Source: CAD feature listing. Evaluate the final solid. Frame: model axes, mm. Give positions to 0.01 mm unless a question says otherwise; leave off trailing zeros. Loops run counter-clockwise (first coordinate to the right, second up) from the corner with the lowest first, then second, coordinate; pieces in that order, holes last. Notation, with made-up numbers: (-2.5, -32) -> (5.5, -32) arc R16 ccw to (5.5, -19) -> close; hole circle Ø10 at (-37.75, 23). An arc over 180 degrees is marked (long way). Put each result on its own line as item: value.
```python
from build123d import *

# Parameters (mm, degrees)
SKETCH2_W           = 170
SKETCH2_H           = 220
SKETCH2_R           = 2.6
SKETCH2_R_2         = 1
SKETCH2_R_3         = 20
BOSS_EXTRUDE1_DEPTH = 3.175


with BuildPart() as part:
    # Sketch2 → Boss-Extrude1 (new body)
    with BuildSketch(Plane(origin=(0, 0, 0), x_dir=(1, 0, 0), z_dir=(0, 1, 0))):
        Rectangle(SKETCH2_W, SKETCH2_H)
        with Locations((-75, 100)):
            Circle(SKETCH2_R, mode=Mode.SUBTRACT)
        with Locations((75, 100)):
            Circle(SKETCH2_R, mode=Mode.SUBTRACT)
        with Locations((75, -100)):
            Circle(SKETCH2_R, mode=Mode.SUBTRACT)
        with Locations((-75, -100)):
            Circle(SKETCH2_R, mode=Mode.SUBTRACT)
        with Locations((-6.954545455, 9)):
            Circle(SKETCH2_R_2, mode=Mode.SUBTRACT)
        with Locations((6.954545455, 9)):
            Circle(SKETCH2_R_2, mode=Mode.SUBTRACT)
        with Locations((6.954545455, -9)):
            Circle(SKETCH2_R_2, mode=Mode.SUBTRACT)
        with Locations((-6.954545455, -9)):
            Circle(SKETCH2_R_2, mode=Mode.SUBTRACT)
        with Locations((0, -48.117139718)):
            Circle(SKETCH2_R_3, mode=Mode.SUBTRACT)
    extrude(amount=BOSS_EXTRUDE1_DEPTH)


solid = part.part
```
(1) Section D-D on y = 1.95. Give the number of separate pieces and of enclosed holes in the cut face, then the cut area to 3 significant figures.
Calculated:
separate pieces: 1
enclosed holes: 9
area: 36,000 mm²
(2) Section A-A on x = -75. Return loops of the section in (y, z) (3 decimals).
Calculated:
outline: (0, -110) -> (3.175, -110) -> (3.175, -102.6) -> (0, -102.6) -> close; (0, -97.4) -> (3.175, -97.4) -> (3.175, 97.4) -> (0, 97.4) -> close; (0, 102.6) -> (3.175, 102.6) -> (3.175, 110) -> (0, 110) -> close
(3) Line query: probe 1 along X at (y, z) = (1.55, 100); probe 2 along Z at (x, y) = (75, 1.2); probe 3 along X at (y, z) = (1.2, 9). Output: solid intervals per line, ascending. Write a range as from..to.
Calculated:
probe 1: x = -85..-77.6, -72.4..72.4, 77.6..85
probe 2: z = -110..-102.6, -97.4..97.4, 102.6..110
probe 3: x = -85..-7.95, -5.95..5.95, 7.95..85
(4) Section B-B on z = 100. Return loops of the section in (x, y) (3 decimals).
Calculated:
outline: (-85, 0) -> (-77.6, 0) -> (-77.6, 3.175) -> (-85, 3.175) -> close; (-72.4, 0) -> (72.4, 0) -> (72.4, 3.175) -> (-72.4, 3.175) -> close; (77.6, 0) -> (85, 0) -> (85, 3.175) -> (77.6, 3.175) -> close
(5) Section C-C on x = 0. Return loops of the section in (y, z) (3 decimals).
Calculated:
outline: (0, -110) -> (3.175, -110) -> (3.175, 28.117) -> (0, 28.117) -> close; (0, 68.117) -> (3.175, 68.117) -> (3.175, 110) -> (0, 110) -> close
(6) Draft query along X for faces 1 (the cylindrical face through (73.084, 1.565, -101.757)), 2 (the flat face through (-1, 0, -2)). Return one class per face: released by +X, released by -X, zero draft, split by the parting line, or undercut.
Calculated:
face 1: undercut
face 2: zero draft
